Build history of the part. All positions in model axes, mm. A direction names the side the tool comes from. Round coordinates to 2 decimals unless told otherwise and drop trailing zeros. Loops run counter-clockwise (first coordinate to the right, second up) from the corner with the lowest first, then second, coordinate; pieces in that order, holes last. Notation, with made-up numbers: (26, 53) - (74, 53) arc R36 ccw to (74, 90) - close; hole circle Ø2 at (47.25, -37). An arc over 180 degrees is marked (long way). Put each result on its own line as item: value. Start each with the question number.
from build123d import *

# Parameters (mm, degrees)
F0_W     = 25.4
F0_H     = 25.4
F1_DEPTH = 25.4
F2_W     = 4.02581
F2_H     = 25.4
F3_DEPTH = 25.4
F4_R     = 1.5875


with BuildPart() as f1:
    # F0 (on Front) → F1 (new body)
    with BuildSketch(Plane.XZ):
        with Locations((12.7, 12.7)):
            Rectangle(F0_W, F0_H)
    extrude(amount=F1_DEPTH)

    # F2 (on face) → F3 (cut)
    with BuildSketch(Plane.XZ.offset(25.4)):
        with Locations((2.012905, 12.7)):
            Rectangle(F2_W, F2_H)
        Polygon((25.4, 25.4), (22.33037, 25.4), (22.33037, 20.32), (10.092464, 20.32), (10.092464, 15.24), (18.617159, 15.24), (18.617159, 10.16), (10.092464, 10.16), (10.092464, 5.08), (22.33037, 5.08), (22.33037, 0), (25.4, 0), align=None)
    extrude(amount=-F3_DEPTH, mode=Mode.SUBTRACT)

    # F4 (on face) → F5 (revolve, cut)
    with BuildSketch(Plane.XZ.offset(25.4)):
        with Locations((19.594045, 23.011442)):
            Circle(F4_R)
    revolve(axis=Axis((19.811029, -25.4, 35.711442), (1, 0, 0)), mode=Mode.SUBTRACT)


solid = f1.part
Item 1: Slice it at D-D (x = 20.25). Give the cut face in (y, z), plus the area to 3 significant figures.
Item 2: Slice it at A-A (x = 12.75). Give the cut face in (y, z), plus the area to 3 significant figures.
Item 3: Two-plate mould, pull along Z, no slides. Class faces 3 (the flat face through (16, -13, 5.08)), 4 (the flat face through (13, -13, 25.4)), 5 (the flat face through (4.026, -13, 13)): pulls with the +Z half, pulls with the -Z half, needs draft (parallel to the pull), parting line crosses it, or undercut.
Item 4: Slice it at B-B (y = -9.5). Give the cut face in (x, z), plus the area to 3 significant figures.
Item 5: Which spindle directions (+Z, -Z, +X, -X, +Y, -Y) get a long thin tool onto all of the face, cutting with end or side? Do faces 1 (the flat face through (14, -13, 10.16)), 2 (the flat face through (22.33, -13, 3)). Say none if no direction does.
Item 6: Drill centre lines: probe 1 along Z at (x, y) = (14.5, -5); probe 2 along Z at (x, y) = (20.5, -12.75); probe 3 along Z at (x, y) = (18.25, -21.5). Where is each one in solid material? Low to high. Write a range as [from, to].
Item 7: Drop flat-ended pins along their axis: pin 1 Ø2.5 at (y, z) = (-11.5, 11.5) entering from +X; pin 2 Ø2 at (y, z) = (-12.5, 17) entering from +X. Give the stop position or say it passes through.
Item 8: Slice it at C-C (z = 7.5). Give the cut face in (x, y).
Computed values:
1. outline: (-25.4, 0) - (0, 0) - (0, 5.08) - (-25.4, 5.08) - close; (-25.4, 20.32) - (0, 20.32) - (0, 25.4) - (-15.72, 25.4) arc R14.15 cw to (-25.4, 21.57) - close; (-25.4, 24.46) arc R11.25 ccw to (-20.89, 25.4) - (-25.4, 25.4) - close
1. area: 235 mm^2
2. outline: (-25.4, 0) - (0, 0) - (0, 5.08) - (-25.4, 5.08) - close; (-25.4, 10.16) - (0, 10.16) - (0, 15.24) - (-25.4, 15.24) - close; (-25.4, 20.32) - (0, 20.32) - (0, 25.4) - (-25.4, 25.4) - close
2. area: 387 mm^2
3. face 3: undercut
3. face 4: pulls with the +Z half
3. face 5: needs draft
4. outline: (4.03, 0) - (22.33, 0) - (22.33, 5.08) - (10.09, 5.08) - (10.09, 10.16) - (18.62, 10.16) - (18.62, 15.24) - (10.09, 15.24) - (10.09, 20.32) - (22.33, 20.32) - (22.33, 25.4) - (4.03, 25.4) - close
4. area: 322 mm^2
5. face 1: +X, +Y, -Y
5. face 2: +Z, -Z, +X, +Y, -Y
6. probe 1: z = [0, 5.08], [10.16, 15.24], [20.32, 25.4]
6. probe 2: z = [0, 5.08], [20.32, 25.4]
6. probe 3: z = [0, 5.08], [10.16, 15.24], [20.32, 22.74], [24.52, 25.4]
7. pin 1: stops at x = 18.62
7. pin 2: stops at x = 10.09
8. outline: (4.03, -25.4) - (10.09, -25.4) - (10.09, 0) - (4.03, 0) - close
